```python
from build123d import *

# Parameters (mm, degrees)
EXTRUDE_1_DEPTH     = 40.8
FILLET_1_R          = 4
CUT_EXTRUDE_1_DEPTH = 2
HOLE_WIZARD_M41_D   = 4.5
CHAMFER_1_SIZE      = 0.5
CHAMFER_1_SIZE2     = 1


with BuildPart() as part:
    # Эскиз1 → Бобышка-Вытянуть1 (new body)
    with BuildSketch(Plane(origin=(0, 0, 0), x_dir=(1, 0, 0), z_dir=(0, 1, 0))):
        Polygon((0, 0), (0, 5), (-11.232050808, 5), (-8.345299462, 0), align=None)
    extrude(amount=EXTRUDE_1_DEPTH)

    # Скругление1
    fillet_1_edges = [part.edges().sort_by_distance(p)[0] for p in [
        (0, 0, -2.5),
        (0, 40.8, -2.5),
    ]]
    fillet(fillet_1_edges, radius=FILLET_1_R)

    # Эскиз4 → Вырез-Вытянуть1 (cut)
    with BuildSketch(Plane.XY):
        with BuildLine():
            Line((-1.672649731, 36.8), (-1.672649731, 26.8))
            ThreePointArc((-1.672649731, 26.8), (-4.172649731, 24.3), (-6.672649731, 26.8))
            Line((-6.672649731, 26.8), (-6.672649731, 36.8))
            ThreePointArc((-6.672649731, 36.8), (-4.172649731, 39.3), (-1.672649731, 36.8))
        make_face()
        with BuildLine():
            Line((-1.672649731, 4), (-1.672649731, 14))
            ThreePointArc((-1.672649731, 14), (-4.172649731, 16.5), (-6.672649731, 14))
            Line((-6.672649731, 14), (-6.672649731, 4))
            ThreePointArc((-6.672649731, 4), (-4.172649731, 1.5), (-1.672649731, 4))
        make_face()
    extrude(amount=-CUT_EXTRUDE_1_DEPTH, mode=Mode.SUBTRACT)

    # Отверстие с зазором M41 (through all)
    with Locations(Plane.XY):
        with Locations((-3.4, 20.4)):
            Hole(HOLE_WIZARD_M41_D / 2)

    # Фаска1
    chamfer_1_edges = [part.edges().sort_by_distance(p)[0] for p in [
        (-11.232050808, 20.4, -5),
    ]]
    chamfer_1_side = [part.faces().sort_by_distance(p)[0] for p in [
        (-5.771423716, 20.4, -5),
    ]]
    chamfer(chamfer_1_edges, length=CHAMFER_1_SIZE, length2=CHAMFER_1_SIZE2, reference=chamfer_1_side[0])


solid = part.part
```
Input: part model. Units: mm. Frame: model coordinates. A direction names the side the tool comes from. Round coordinates to 2 decimals unless told otherwise and drop trailing zeros. Loops run counter-clockwise (first coordinate to the right, second up) from the corner with the lowest first, then second, coordinate; pieces in that order, holes last. Notation, with made-up numbers: M 28,49.5 L 85,49.5 A25 ccw 85,78.5 Z; hole C 48.5,-15 d1. An arc over 180 degrees is marked long. Answer in a Markdown table with one row per item. Add a question column.
1. Section B-B (x = -5.25). Output: boundary loops of the cut face in (y, z), and give its area (3 significant figures).
2. Ray query, probe 1 along Y at (x, z) = (-3.4, -1.75); probe 2 along Y at (x, z) = (-5.75, -1.3); probe 3 along X at (y, z) = (26.5, -0.5). Return the intervals inside material, ascending.
3. Mould query, pull axis X, two halves, no side actions, for faces 3 (the face through (-4.2, 1.5, -1)), 4 (the face through (-4, 9, -2)), 5 (the face through (-7, 0, -3)), 6 (the face through (0, 20, -2)). Classes: released by +X, released by -X, zero draft, split by the parting line, or undercut.
4. Section A-A (y = 20.4). Output: boundary loops of the cut face in (x, z).
5. Set-up query: faces 1 (the face through (-1.141, 1.203, -2.535)), 2 (the face through (-6.673, 32, -1)). Return all of +Z, -Z, +X, -X, +Y, -Y with unobstructed straight access to the full face (end or side cutting, diameter ignored); none if empty.
6. Section D-D (y = 35.5). Output: boundary loops of the cut face in (x, z).
7. Contact query for flat-ended pins moving along their axis: pin 1 (2 mm diameter, centred on x = -2, z = -1, fed in from -Y); pin 2 (1.6 mm diameter, centred on y = 10, z = -1, fed in from -X); pin 3 (3 mm diameter, centred on x = -5, y = 27.5, fed in from +Z); pin 4 (3.5 mm diameter, centred on x = -3.4, y = 20.4, fed in from +Z). Output: stop coordinate, or through.
8. Section C-C (z = -2.75). Output: boundary loops of the cut face in (x, y).
Values follow:
| question | item | result |
|---|---|---|
| 1 | outline | M 0,-5 L 19.12,-5 L 19.12,0 L 16.26,0 L 16.26,-2 L 1.74,-2 L 1.74,0 L 0,0 Z; M 21.68,-5 L 40.8,-5 L 40.8,0 L 39.06,0 L 39.06,-2 L 24.54,-2 L 24.54,0 L 21.68,0 Z |
| 1 | area | 133 mm^2 |
| 2 | probe 1 | 0.05 to 1.62, 16.38 to 18.15, 22.65 to 24.42, 39.18 to 40.75 |
| 2 | probe 2 | 0 to 2.06, 15.94 to 24.86, 38.74 to 40.8 |
| 2 | probe 3 | -8.63 to -6.65, -1.69 to 0 |
| 3 | face 3 | undercut |
| 3 | face 4 | undercut |
| 3 | face 5 | zero draft |
| 3 | face 6 | released by +X |
| 4 | outline | M -10.73,-5 L -5.65,-5 L -5.65,0 L -8.35,0 L -10.73,-4.13 Z; M -1.15,-5 L 0,-5 L 0,0 L -1.15,0 Z |
| 5 | face 1 | +Z, -Z, +X, -Y |
| 5 | face 2 | +Z |
| 6 | outline | M -10.73,-5 L 0,-5 L 0,0 L -1.67,0 L -1.67,-2 L -6.67,-2 L -6.67,0 L -8.35,0 L -10.73,-4.13 Z |
| 7 | pin 1 | y = 0.13 |
| 7 | pin 2 | x = -9.38 |
| 7 | pin 3 | z = -2 |
| 7 | pin 4 | through |
| 8 | outline | M -9.93,0 L -4,0 A4 ccw 0,4 L 0,36.8 A4 ccw -4,40.8 L -9.93,40.8 Z; hole C -3.4,20.4 d4.5 |
